Model file for the job. Use its own axes, mm. A direction names the side the tool comes from. Round coordinates to 2 decimals unless told otherwise and drop trailing zeros. Loops run counter-clockwise (first coordinate to the right, second up) from the corner with the lowest first, then second, coordinate; pieces in that order, holes last. Notation, with made-up numbers: M 74,-9 L 120,-9 A15 cw 120,-5 Z; hole C 3,-0.75 d1. An arc over 180 degrees is marked long. Answer in a Markdown table with one row per item.
from build123d import *

# Parameters (mm, degrees)
SKETCH007_W        = 150
SKETCH007_H        = 110
PAD002_DEPTH       = 12
SKETCH008_W        = 145.5
SKETCH008_H        = 105.5
POCKET004_DEPTH    = 10
POCKET005_DEPTH    = 5
POLARPATTERN_COUNT = 9


with BuildPart() as part:
    # Sketch007 → Pad002 (new body)
    with BuildSketch(Plane.XY):
        Rectangle(SKETCH007_W, SKETCH007_H)
    extrude(amount=PAD002_DEPTH)

    # Sketch008 (on Face6 of Pad002) → Pocket004 (cut)
    with BuildSketch(Plane.XY.offset(12)):
        Rectangle(SKETCH008_W, SKETCH008_H)
    extrude(amount=-POCKET004_DEPTH, mode=Mode.SUBTRACT)

    # Sketch009 (on Face11 of Pocket004) → Pocket005 (cut)
    with BuildSketch(Plane.XY.offset(2)):
        with BuildLine():
            Line((-0.935974, 47.157331), (0.935974, 47.157331))
            ThreePointArc((4.532255, 43.120312), (3.639248, 45.945137), (0.935974, 47.157331))
            Line((4.532255, 43.120312), (0, 4.003277))
            Line((0, 4.003277), (-4.532255, 43.120312))
            ThreePointArc((-0.935974, 47.157331), (-3.639248, 45.945137), (-4.532255, 43.120312))
        make_face()
    pocket005 = extrude(amount=-POCKET005_DEPTH, mode=Mode.SUBTRACT)

    # PolarPattern: Pocket005 ×9 about axis
    polarpattern_axis = Axis((0, 0, 2), (0, 0, 1))
    for i in range(1, POLARPATTERN_COUNT):
        add(pocket005.rotate(polarpattern_axis, i * 360 / POLARPATTERN_COUNT), mode=Mode.SUBTRACT)


solid = part.part
1. Saw through at B-B (y = -14). Write the cut outline in (x, z), and give its area (3 significant figures).
Verdict:
| item | result |
|---|---|
| outline | M -75,0 L -31.21,0 L -31.21,2 L -72.75,2 L -72.75,12 L -75,12 Z; M -19.62,0 L -6.5,0 L -6.5,2 L -19.62,2 Z; M -3.81,0 L 3.81,0 L 3.81,2 L -3.81,2 Z; M 6.5,0 L 19.62,0 L 19.62,2 L 6.5,2 Z; M 31.21,0 L 75,0 L 75,12 L 72.75,12 L 72.75,2 L 31.21,2 Z |
| area | 288 mm² |
2. Saw through at D-D (y = -32.5). Write the cut outline in (x, z), and give its area (3 significant figures).
Verdict:
| item | result |
|---|---|
| outline | M -75,0 L -15.77,0 L -15.77,2 L -72.75,2 L -72.75,12 L -75,12 Z; M -8.21,0 L 8.21,0 L 8.21,2 L -8.21,2 Z; M 15.77,0 L 75,0 L 75,12 L 72.75,12 L 72.75,2 L 15.77,2 Z |
| area | 315 mm² |
3. Pin check, flat tip, straight feed: pin 1 (12 mm diameter, centred on x = -24.5, y = 2.5, fed in from +Z). Stop position of the tip, or through.
Verdict:
| item | result |
|---|---|
| pin 1 | stops at z = 2 |
4. Mould opens along Y. For faces 1 (the flat face through (-1, -55, 6)), 2 (the flat face through (22.546, 6.244, 1.014)), 3 (the flat face through (-1, 1, 0)) say: +Y half, -Y half, draft (parallel to the pull), parting line (faces both ways), or undercut.
Verdict:
| item | result |
|---|---|
| face 1 | -Y half |
| face 2 | undercut |
| face 3 | draft |
5. Wall check: probe 1 along X at (y, z) = (29, 2.75); probe 2 along X at (y, z) = (16.5, 1.25); probe 3 along X at (y, z) = (-12.5, 1.5). Give the ranges that are in metal, low to high.
Verdict:
| item | result |
|---|---|
| probe 1 | x = -75 to -72.75, 72.75 to 75 |
| probe 2 | x = -75 to -16.78, -11.43 to -1.45, 1.45 to 11.43, 16.78 to 75 |
| probe 3 | x = -75 to -27.74, -17.6 to -5.75, -3.45 to 3.45, 5.75 to 17.6, 27.74 to 75 |
6. Saw through at A-A (z = 6.25). Write the cut outline in (x, y), and give its area (3 significant figures).
Verdict:
| item | result |
|---|---|
| outline | M -75,-55 L 75,-55 L 75,55 L -75,55 Z; hole M -72.75,-52.75 L 72.75,-52.75 L 72.75,52.75 L -72.75,52.75 Z |
| area | 1,150 mm² |
7. Saw through at C-C (x = -53.5). Write the cut outline in (y, z).
Verdict:
| item | result |
|---|---|
| outline | M -55,0 L 55,0 L 55,12 L 52.75,12 L 52.75,2 L -52.75,2 L -52.75,12 L -55,12 Z |
8. Tool access for faces 4 (the flat face through (0, 53, 12)), 5 (the flat face through (-1, 52.75, 7)), 6 (the cylindrical face through (3.67, 45.91, 1.01)): list every direction of +Z, -Z, +X, -X, +Y, -Y with a clear straight run to the whole face (end or side of a thin tool).
Verdict:
| item | result |
|---|---|
| face 4 | +Z, +X, -X, +Y, -Y |
| face 5 | +Z |
| face 6 | +Z, -Z |
